Work out the finished part from the listing and answer in its coordinate system (mm). Face numbers are marked on the shaded views. A direction names the side the tool comes from. Give positions to 0.01 mm unless a question says otherwise; leave off trailing zeros. Loops run counter-clockwise (first coordinate to the right, second up) from the corner with the lowest first, then second, coordinate; pieces in that order, holes last.
Autodesk Inventor part; units mm, degrees
ref_plane "YZ Plane" through (0, 0, 0) normal (1, 0, 0) x (0, 1, 0)
ref_plane "XZ Plane" through (0, 0, 0) normal (0, 1, 0) x (-1, 0, 0)
ref_plane "XY Plane" through (0, 0, 0) normal (0, 0, 1) x (1, 0, 0)
sketch "Эскиз1" plane through (0, 0, 0) normal (1, 0, 0) x (0, 1, 0)
  line L0 (16.7932, 4.1754) -> (-3.2068, 4.1754)
  line L1 (-3.2068, 4.1754) -> (-3.2068, 24.1754)
  line L2 (-3.2068, 24.1754) -> (16.7932, 24.1754)
  line L3 (16.7932, 24.1754) -> (16.7932, 4.1754)
  line L4 (-1.7068, 5.6754) -> (15.2932, 5.6754)
  line L5 (15.2932, 5.6754) -> (15.2932, 22.6754)
  line L6 (15.2932, 22.6754) -> (-1.7068, 22.6754)
  line L7 (-1.7068, 22.6754) -> (-1.7068, 5.6754)
  point P0 (6.7932, 5.6754)
  point P1 (6.7932, 4.1754)
  dimension "d1" = 20
  dimension "d2" = 1.5
  dimension "d3" = 1.5
extrude "Выдавливание1" add sketch "Эскиз1" against normal blind 20
properties part number "arm"
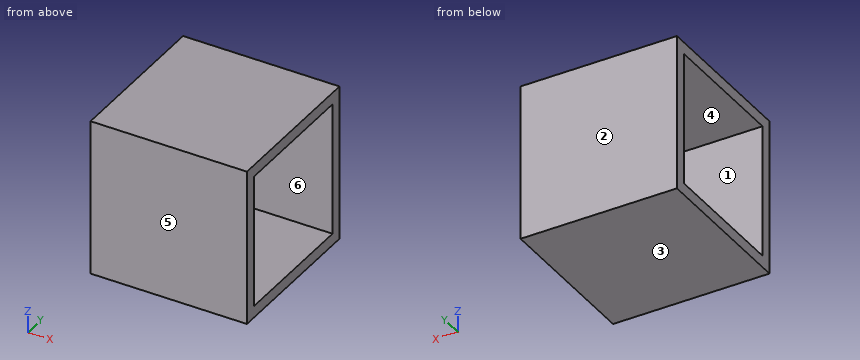
Q1. Which of the six approach directions +Z, -Z, +X, -X, +Y, -Y give full straight-line access (tool end or side, diameter ignored) to the marked faces 1 and 2?
Q2. Determine the mould class of the marked faces 3, 4, 5 and 6 for opening direction Y: +Y half, -Y half, draft (parallel to the pull), parting line (faces both ways), or undercut.
Q3. Section B-B on z = 21.5 is taken. Give the vertices of the cut face in (x, y), plus the area to 3 significant figures.
Q4. Section C-C on x = -16.5 is taken. Give the vertices of the cut face in (y, z), plus the area to 3 significant figures.
Q5. Section A-A on y = -1.25 is taken. Give the vertices of the cut face in (x, z), plus the area to 3 significant figures.
Q6. Consider line 1 along Y through (x, z) = (-4.25, 12); line 2 along Z through (x, y) = (-12, 7.5). Determine where each line is inside the solid, lowest interval first.
Check result:
1. face 1: +X, -X
1. face 2: +Z, -Z, +X, -X, +Y
2. face 3: draft
2. face 4: undercut
2. face 5: -Y half
2. face 6: undercut
3. outline: (-20, -3.21) - (0, -3.21) - (0, -1.71) - (-20, -1.71) - close; (-20, 15.29) - (0, 15.29) - (0, 16.79) - (-20, 16.79) - close
3. area: 60.0 mm2
4. outline: (-3.21, 4.18) - (16.79, 4.18) - (16.79, 24.18) - (-3.21, 24.18) - close; hole (-1.71, 5.68) - (15.29, 5.68) - (15.29, 22.68) - (-1.71, 22.68) - close
4. area: 111 mm2
5. outline: (-20, 4.18) - (0, 4.18) - (0, 5.68) - (-20, 5.68) - close; (-20, 22.68) - (0, 22.68) - (0, 24.18) - (-20, 24.18) - close
5. area: 60.0 mm2
6. line 1: y = -3.21 to -1.71, 15.29 to 16.79
6. line 2: z = 4.18 to 5.68, 22.68 to 24.18
